Autodesk Inventor part; units mm, degrees
ref_plane "YZ Plane" through (0, 0, 0) normal (1, 0, 0) x (0, 1, 0)
ref_plane "XZ Plane" through (0, 0, 0) normal (0, 1, 0) x (-1, 0, 0)
ref_plane "XY Plane" through (0, 0, 0) normal (0, 0, 1) x (1, 0, 0)
sketch "スケッチ1" plane through (0, 0, 0) normal (0, 0, 1) x (1, 0, 0)
  line L0 (5.5, -5.5) -> (-5.5, -5.5)
  line L1 (-5.5, -5.5) -> (-5.5, 5.5)
  line L2 (-5.5, 5.5) -> (5.5, 5.5)
  line L3 (5.5, 5.5) -> (5.5, -5.5)
  line L4 (5.5, -5.5) -> (-5.5, 5.5) construction
  line L5 (-5.5, -5.5) -> (5.5, 5.5) construction
  line L6 (7.5, -7.5) -> (-7.5, -7.5)
  line L7 (-7.5, -7.5) -> (-7.5, 7.5)
  line L8 (-7.5, 7.5) -> (7.5, 7.5)
  line L9 (7.5, 7.5) -> (7.5, -7.5)
  line L10 (7.5, -7.5) -> (-7.5, 7.5) construction
  line L11 (-7.5, -7.5) -> (7.5, 7.5) construction
  point P0 (0, 0)
  dimension "d0" = 11
  dimension "d1" = 11
  dimension "d2" = 2
extrude "押し出し1" add sketch "スケッチ1" along normal blind 14
sketch "スケッチ2" plane through (0, 0, 14) normal (0, 0, 1) x (1, 0, 0)
  line L0 (-7.5, 7.5) -> (-7.5, -7.5)
  line L1 (-7.5, -7.5) -> (-14.5, -7.5)
  line L2 (-14.5, -7.5) -> (-14.5, -4.5)
  line L3 (-14.5, -4.5) -> (-7.5, -4.5)
  line L4 (-7.5, -4.5) -> (-7.5, -7.5)
  arc A0 (-14.5, -4.5) -> (-7.5, 7.5) centre (-21.2857, 7.5) ccw
  point P0 (0, 0)
  dimension "d5" = 7
  dimension "d6" = 3
extrude "押し出し2" add sketch "スケッチ2" against normal up to surface (14 mm away)
sketch "スケッチ3" plane through (7.5, 7.5, 14) normal (0, 1, 0) x (1, 0, 0)
  circle A0 centre (-7.5, 7) radius 1.4
  line L0 (0, 14) -> (0, 0)
  line L1 (0, 14) -> (-15, 14)
  point P0 (-7.5, 14)
  point P1 (0, 7)
  point P2 (-7.5, 14)
  dimension "d9" = 2.8
extrude "押し出し3" cut sketch "スケッチ3" against normal up to surface (2 mm away)
sketch "スケッチ4" plane through (7.5, -7.5, 0) normal (0, -1, 0) x (1, 0, 0)
  line L0 (-6, 12) -> (-4, 12)
  line L1 (-4, 12) -> (-4, 2)
  line L2 (-4, 2) -> (-6, 2)
  line L3 (-6, 2) -> (-6, 12)
  line L4 (-10, 8) -> (0, 8)
  line L5 (0, 8) -> (0, 6)
  line L6 (0, 6) -> (-10, 6)
  line L7 (-10, 6) -> (-10, 8)
  line L8 (0, 0) -> (0, 14)
  point P0 (-7.5, 0)
  point P1 (0, 7)
  point P2 (0, 7)
  point P3 (-5, 12)
  point P4 (-5, 8)
  point P5 (-6, 7)
  point P6 (-10, 7)
  point P7 (-6, 8)
  point P8 (-6, 6)
  point P9 (-4, 6)
  point P10 (-4, 8)
  dimension "d12" = 10
  dimension "d13" = 2
extrude "押し出し4" add sketch "スケッチ4" along normal blind 5
sketch "スケッチ5" plane through (7.5, 7.5, 14) normal (0, 1, 0) x (1, 0, 0)
  line L0 (-15.3, 8.3568) -> (-15.3, 5.6432)
  line L1 (-15.3, 5.6432) -> (-17.65, 4.2865)
  line L2 (-17.65, 4.2865) -> (-20, 5.6432)
  line L3 (-20, 5.6432) -> (-20, 8.3568)
  line L4 (-20, 8.3568) -> (-17.65, 9.7135)
  line L5 (-17.65, 9.7135) -> (-15.3, 8.3568)
  circle A0 centre (-17.65, 7) radius 1.6
  line L6 (-22, 0) -> (-22, 14)
  point P0 (-7.5, 14)
  point P1 (-20, 7)
  point P2 (-22, 7)
  dimension "d16" = 4.7
  dimension "d17" = 3.2
  dimension "d24" = 2
extrude "押し出し5" cut sketch "スケッチ5" against normal through all contours A0
extrude "押し出し6" cut sketch "スケッチ5" against normal up to surface (13 mm away) contours L0 L1 L2 L3 L4 L5 | A0
properties part number "position_setter_normal"
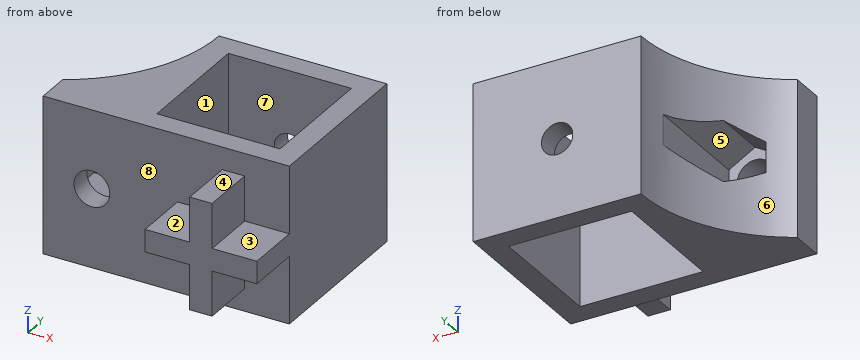
Input: part model. Units: mm. Frame: model coordinates. Face numbers are marked on the shaded views. A direction names the side the tool comes from. Round coordinates to 2 decimals unless told otherwise and drop trailing zeros. Loops run counter-clockwise (first coordinate to the right, second up) from the corner with the lowest first, then second, coordinate; pieces in that order, holes last. Notation, with made-up numbers: M 41,51.5 L 100,51.5 A20 ccw 100,68.5 Z; hole C 15,83.5 d3. An arc over 180 degrees is marked long. Answer in a Markdown table with one row per item. Add a question column.
1. Contact query for flat-ended pins moving along their axis: pin 1 (1.6 mm diameter, centred on y = -9, z = 6.5, fed in from -X); pin 2 (2 mm diameter, centred on y = -11, z = 11, fed in from +X); pin 3 (2.5 mm diameter, centred on x = -10, z = 6.5, fed in from +Y). Output: stop coordinate, or through.
2. Section D-D (x = -5). Output: boundary loops of the cut face in (y, z), and give its area (3 significant figures).
3. Set-up query: the marked faces 1, 2, 3, 4 and 5. Return all of +Z, -Z, +X, -X, +Y, -Y with unobstructed straight access to the full face (end or side cutting, diameter ignored); none if empty.
4. Ray query, probe 1 along Z at (x, y) = (0, 6.9); probe 2 along Y at (x, z) = (1, 3); probe 3 along Z at (x, y) = (-10.15, -6). Return the intervals inside material, ascending.
5. Mould query, pull axis X, two halves, no side actions, for the marked faces 6, 7 and 8. Classes: released by +X, released by -X, zero draft, split by the parting line, or undercut.
6. Section B-B (y = -3.5). Output: boundary loops of the cut face in (x, z), and give its area (3 significant figures).
7. Section C-C (z = 10). Output: boundary loops of the cut face in (x, y).
8. Section A-A (x = 0). Output: boundary loops of the cut face in (y, z), and give its area (3 significant figures).
Values follow:
| question | item | result |
|---|---|---|
| 1 | pin 1 | x = -2.5 |
| 1 | pin 2 | x = 3.5 |
| 1 | pin 3 | y = -5.5 |
| 2 | outline | M -7.5,0 L -5.5,0 L -5.5,14 L -7.5,14 Z; M 5.5,0 L 7.5,0 L 7.5,14 L 5.5,14 Z |
| 2 | area | 56.0 mm^2 |
| 3 | face 1 | +Z, -Z |
| 3 | face 2 | +Z, -X, -Y |
| 3 | face 3 | +Z, +X, -Y |
| 3 | face 4 | +Z, +X, -X, -Y |
| 3 | face 5 | +Y |
| 4 | probe 1 | 0 to 5.6, 8.4 to 14 |
| 4 | probe 2 | -7.5 to -5.5, 5.5 to 7.5 |
| 4 | probe 3 | 0 to 5.4, 8.6 to 14 |
| 5 | face 6 | released by -X |
| 5 | face 7 | undercut |
| 5 | face 8 | zero draft |
| 6 | outline | M -12.98,0 L -5.5,0 L -5.5,14 L -12.98,14 Z; M 5.5,0 L 7.5,0 L 7.5,14 L 5.5,14 Z; hole M -12.5,5.64 L -10.15,4.29 L -7.8,5.64 L -7.8,8.36 L -10.15,9.71 L -12.5,8.36 Z |
| 6 | area | 114 mm^2 |
| 7 | outline | M -14.5,-7.5 L 1.5,-7.5 L 1.5,-12.5 L 3.5,-12.5 L 3.5,-7.5 L 7.5,-7.5 L 7.5,7.5 L -7.5,7.5 A13.79 cw -14.5,-4.5 Z; hole M -5.5,-5.5 L 5.5,-5.5 L 5.5,5.5 L -5.5,5.5 Z |
| 8 | outline | M -12.5,6 L -7.5,6 L -7.5,0 L -5.5,0 L -5.5,14 L -7.5,14 L -7.5,8 L -12.5,8 Z; M 5.5,0 L 7.5,0 L 7.5,5.6 L 5.5,5.6 Z; M 5.5,8.4 L 7.5,8.4 L 7.5,14 L 5.5,14 Z |
| 8 | area | 60.4 mm^2 |
